Here's the drawing with two shaded views (mm, measured from the low corner). I have some questions. A direction names the side the tool comes from. Round coordinates to 2 decimals unless told otherwise and drop trailing zeros. Loops run counter-clockwise (first coordinate to the right, second up) from the corner with the lowest first, then second, coordinate; pieces in that order, holes last.
(1) I want a section at B-B on z = 1.5. Write out the boundary of the cut face in (x, y) (1 decimal), plus the area to 3 significant figures.
(2) If I drill on line 1 along X through (y, z) = (7.5, 2.75) (1 decimal); line 2 along Y through (x, z) = (36, 5.5); line 3 along X through (y, z) = (17, 2.75) (1 decimal), over which ranges is the centre line in solid material (lowest first)?
(3) Will these pins go through, and if not, where does the flat tip stop? pin 1 Ø6 at (x, y) = (13.5, 14.5) entering from -Z; pin 2 Ø3 at (x, z) = (41, 10.5) entering from -Y; pin 3 Ø2.5 at (x, z) = (49.66, 20.52) entering from +Y.
(4) Thinking about a two-plate mould opening in Z: for the marked faces 1, 2, 3 and 4, which applies, released by +Z, released by -Z, zero draft, split by the parting line, or undercut?
(5) Which directions (+Z, -Z, +X, -X, +Y, -Y) give clear straight access to the entire face, cutting with the end or side of a thin tool? Please do the marked faces 5 and 6.
(6) I want a section at C-C on y = 11.75. Write out the boundary of the cut face in (x, z) (1 decimal), plus the area to 3 significant figures.
(7) I want a section at D-D on z = 9. Write out the boundary of the cut face in (x, y), plus the area to 3 significant figures.
(8) I want a section at A-A on y = 5.5. Write out the boundary of the cut face in (x, z) (1 decimal).
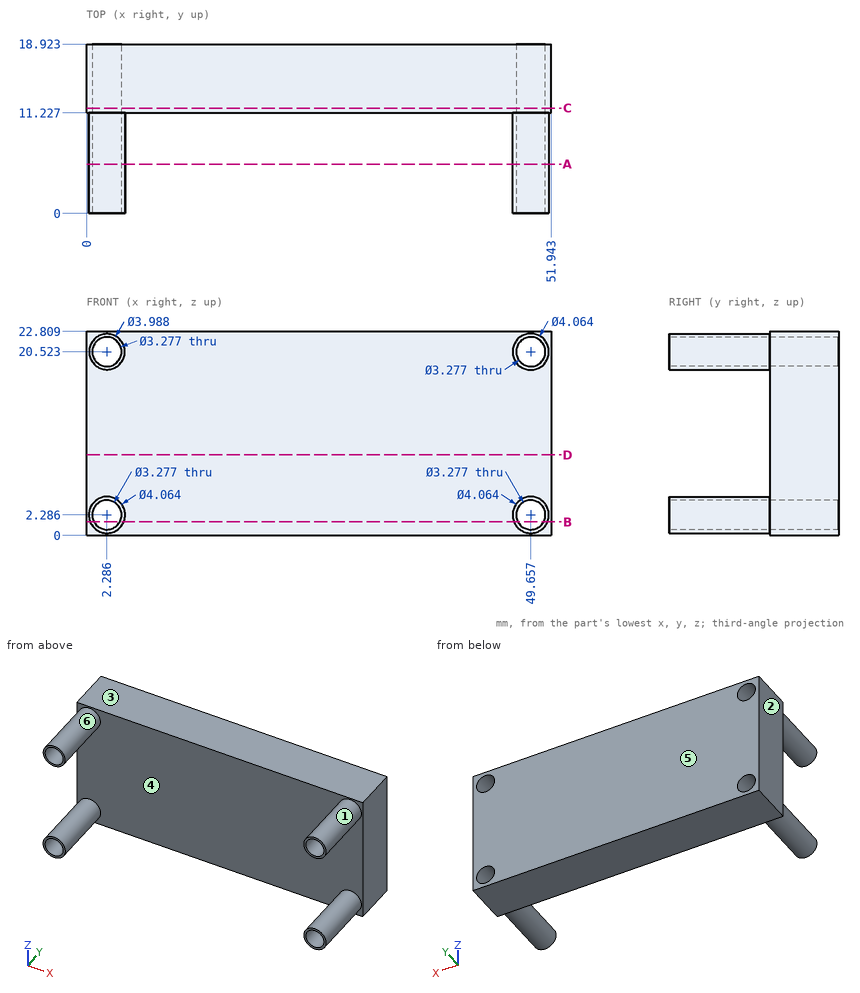
Filled sheet:
1. outline: (0, 11.2) - (0.4, 11.2) - (0.4, 0) - (0.8, 0) - (0.8, 18.9) - (0, 18.9) - close; (3.7, 0) - (4.2, 0) - (4.2, 11.2) - (47.8, 11.2) - (47.8, 0) - (48.2, 0) - (48.2, 18.9) - (3.7, 18.9) - close; (51.1, 0) - (51.5, 0) - (51.5, 11.2) - (51.9, 11.2) - (51.9, 18.9) - (51.1, 18.9) - close
1. area: 375 mm2
2. line 1: x = 0.3 to 0.7, 3.9 to 4.3, 47.7 to 48.1, 51.2 to 51.6
2. line 2: y = 11.23 to 18.92
2. line 3: x = 0 to 0.7, 3.9 to 48.1, 51.2 to 51.9
3. pin 1: stops at z = 0
3. pin 2: stops at y = 11.23
3. pin 3: passes through
4. face 1: undercut
4. face 2: zero draft
4. face 3: released by +Z
4. face 4: undercut
5. face 5: +Z, -Z, +X, -X, +Y
5. face 6: -Y
6. outline: (0, 0) - (51.9, 0) - (51.9, 22.8) - (0, 22.8) - close; hole circle Ø3.3 at (2.3, 2.3); hole circle Ø3.3 at (2.3, 20.5); hole circle Ø3.3 at (49.7, 2.3); hole circle Ø3.3 at (49.7, 20.5)
6. area: 1,150 mm2
7. outline: (0, 11.23) - (51.94, 11.23) - (51.94, 18.92) - (0, 18.92) - close
7. area: 400 mm2
8. outline: circle Ø4.1 at (2.3, 2.3); circle Ø4 at (2.3, 20.5); circle Ø4.1 at (49.7, 2.3); circle Ø4.1 at (49.7, 20.5); hole circle Ø3.3 at (2.3, 2.3); hole circle Ø3.3 at (2.3, 20.5); hole circle Ø3.3 at (49.7, 2.3); hole circle Ø3.3 at (49.7, 20.5)
